Verification items for the finished model (mm, model axes). A direction names the side the tool comes from. Round coordinates to 2 decimals unless told otherwise and drop trailing zeros. Order: outer loops, then holes, each group sorted by start corner. A loop starts at its lowest first (then second) coordinate and runs counter-clockwise, first axis right, second up. Notation, with made-up numbers: M 50.5,-25.5 L 106.5,-25.5 A16 cw 106.5,-9.5 Z; hole C -17.5,45 d8. An arc over 180 degrees is marked long. Use one line per item in the form item = value. Start each with the question number.
Item 1: Thickness scan on probe 1 along Y at (x, z) = (63.5, 1.75) (3 decimals); probe 2 along Z at (x, y) = (107, 0.75) (3 decimals); probe 3 along X at (y, z) = (1, -1.5) (3 decimals). Record the ranges inside material, lowest first. Write a range as [from, to].
Item 2: Release check for a two-part mould opening along Y. For faces 3 (the flat face through (2.425, 0.089, -0.75)), 4 (the flat face through (75, 3.175, 2)), 5 (the flat face through (75, -6.35, 0)) record: +Y half, -Y half, draft (parallel to the pull), parting line (faces both ways), or undercut.
Item 3: Cross-section at B-B on x = 89.5. Enter the section's corners in (y, z) (3 decimals), then the cut area to 3 significant figures.
Item 4: Tool access check on faces 1 (the flat face through (75, 0, 0)), 2 (the flat face through (75, 6.35, 0)). Record the directions out of +Z, -Z, +X, -X, +Y, -Y that give a thin tool (end or side, any length) a straight path to the whole face; none if there is none.
Item 5: Cross-section at A-A on z = 2. Enter the section's corners in (x, y) (3 decimals), then the cut area to 3 significant figures.
Item 6: Go/stop test with flat-tipped pins: pin 1 Ø1.9 at (x, y) = (78.5, 0) entering from +Z; pin 2 Ø1.5 at (y, z) = (5, 0.5) entering from -X (3 decimals). Record where each tip stops, or that it passes through.
Item 7: Cross-section at C-C on y = 0.75. Enter the section's corners in (x, z) (3 decimals).
from build123d import *

# Parameters (mm, degrees)
F1_DEPTH = 152.4
F3_DEPTH = 6.35


with BuildPart() as f1:
    # F0 (on Right) → F1 (new body)
    with BuildSketch(Plane.YZ):
        Polygon((6.35, -3.175), (6.35, 3.175), (3.175, 3.175), (3.175, 0), (-3.175, 0), (-3.175, 3.175), (-6.35, 3.175), (-6.35, -3.175), align=None)
    extrude(amount=F1_DEPTH)

    # F2 (on Front) → F3 (cut, symmetric)
    with BuildSketch(Plane.XZ):
        Polygon((0, 3.175), (0, -3.175), (6.35, 3.175), align=None)
        Polygon((146.05, 3.175), (152.4, -3.175), (152.4, 3.175), align=None)
    extrude(amount=F3_DEPTH, both=True, mode=Mode.SUBTRACT)


solid = f1.part
Output values:
q1.probe_1 = [-6.35, -3.175], [3.175, 6.35]
q1.probe_2 = [-3.175, 0]
q1.probe_3 = [1.675, 150.725]
q2.face_3 = draft
q2.face_4 = undercut
q2.face_5 = -Y half
q3.outline = M -6.35,-3.175 L 6.35,-3.175 L 6.35,3.175 L 3.175,3.175 L 3.175,0 L -3.175,0 L -3.175,3.175 L -6.35,3.175 Z
q3.area = 60.5 mm2
q4.face_1 = +Z, +X, -X
q4.face_2 = +Z, -Z, +X, -X, +Y
q5.outline = M 5.175,-6.35 L 147.225,-6.35 L 147.225,-3.175 L 5.175,-3.175 Z; M 5.175,3.175 L 147.225,3.175 L 147.225,6.35 L 5.175,6.35 Z
q5.area = 902 mm2
q6.pin_1 = 0
q6.pin_2 = 2.925
q7.outline = M 0,-3.175 L 152.4,-3.175 L 149.225,0 L 3.175,0 Z
